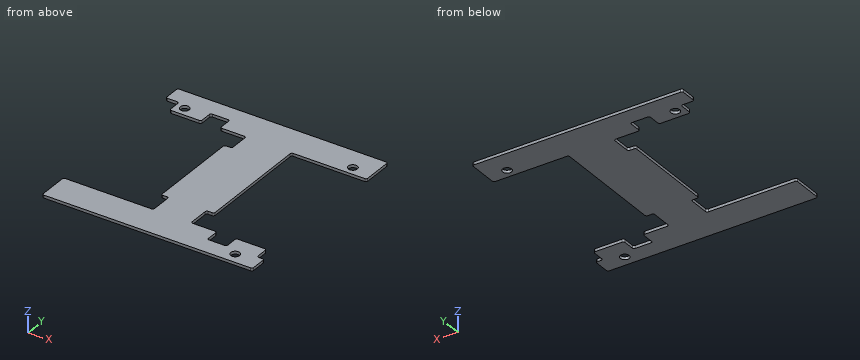
Autodesk Inventor part; units mm, degrees
ref_plane "YZ Plane" through (0, 0, 0) normal (1, 0, 0) x (0, 1, 0)
ref_plane "XZ Plane" through (0, 0, 0) normal (0, 1, 0) x (-1, 0, 0)
ref_plane "XY Plane" through (0, 0, 0) normal (0, 0, 1) x (1, 0, 0)
sketch "Sketch1" plane through (0, 0, 0) normal (0, 0, 1) x (1, 0, 0)
  line L0 (13.7023, 4) -> (22.3525, 4)
  line L1 (22.3525, 0) -> (59.3371, 0)
  line L2 (59.3371, 0) -> (59.3371, 9.3)
  line L3 (59.3371, 9.3) -> (0, 9.3)
  line L4 (0, 4) -> (0, 9.3)
  line L5 (2.4551, 0) -> (13.7023, 0)
  line L6 (0, -38.4) -> (39.318, -38.4)
  line L7 (0, -38.4) -> (0, -47.7)
  line L8 (0, -47.7) -> (59.3371, -47.7)
  line L9 (59.3371, -42.4) -> (59.3371, -47.7)
  line L10 (59.3371, -42.4) -> (58.882, -42.4)
  line L11 (58.882, -42.4) -> (58.882, -38.4)
  line L12 (47.6348, -38.4) -> (58.882, -38.4)
  line L13 (47.6348, -42.4) -> (39.318, -42.4)
  line L14 (39.0735, -33.15) -> (39.0735, -5.25)
  line L15 (39.0735, -5.25) -> (39.9371, -5.25)
  line L16 (39.9371, -5.25) -> (39.9371, -33.15)
  line L17 (39.9371, -33.15) -> (39.0735, -33.15)
  line L18 (22.2636, -5.25) -> (22.2636, -33.15)
  line L19 (22.2636, -33.15) -> (21.4, -33.15)
  line L20 (21.4, -33.15) -> (21.4, -5.25)
  line L21 (21.4, -5.25) -> (22.2636, -5.25)
  line L22 (21.4, 0) -> (21.4, -38.4)
  line L23 (39.9371, -38.4) -> (39.9371, 0)
  line L24 (39.9371, 0) -> (62.3371, 0)
  line L25 (59.1371, 9.1) -> (59.1371, 0.2)
  line L26 (59.1371, 0.2) -> (38.0735, 0.2)
  line L27 (38.0735, 0.2) -> (38.0735, -6.25)
  line L28 (38.0735, -6.25) -> (38.0735, -6.25)
  line L29 (38.0735, -6.25) -> (38.0735, -32.15)
  line L30 (35.9371, -32.15) -> (35.9371, -38.6)
  line L31 (59.1371, -42.6) -> (59.1371, -47.5)
  line L32 (59.1371, -47.5) -> (46.1371, -47.5)
  line L33 (0.2, -47.5) -> (0.2, -38.6)
  line L34 (0.2, -38.6) -> (25.4, -38.6)
  line L35 (25.4, -38.6) -> (25.4, -32.15)
  line L36 (25.4, -32.15) -> (23.2636, -32.15)
  line L37 (23.2636, -32.15) -> (23.2636, -5.75)
  line L38 (23.2636, -5.75) -> (25.4, -5.75)
  line L39 (25.4, -5.75) -> (25.4, 0.2)
  line L40 (0.2, 4.2) -> (0.2, 8.5299)
  line L41 (38.0735, -32.15) -> (35.9371, -32.15)
  line L42 (12.7424, 4.2) -> (12.7424, 0.2)
  line L43 (12.7424, 0.2) -> (3.912, 0.2)
  line L44 (3.912, 0.2) -> (3.912, 4.2)
  line L45 (3.912, 4.2) -> (0.2, 4.2)
  line L46 (59.1371, -42.6) -> (57.125, -42.6)
  line L47 (57.125, -42.6) -> (57.125, -38.6)
  line L48 (57.125, -38.6) -> (48.5947, -38.6)
  line L49 (48.5947, -38.6) -> (48.5947, -42.6)
  line L50 (39.318, -42.4) -> (39.318, -38.4)
  line L51 (47.6348, -38.4) -> (47.6348, -42.4)
  line L52 (22.3525, 4) -> (22.3525, 0)
  spline S0 degree 2 poles (41.0471, 11.3) (40.5342, 11.2191) (40.0213, 11.3) knots 0 0 0 0.102903 0.102903 0.102903 weights 1 1.01269 1
  line L53 (0, 11.3) -> (40.0213, 11.3)
  line L54 (0, 9.3) -> (0, 11.3)
  line L55 (0, 9.3) -> (46.3371, 9.3)
  line L56 (46.3371, 9.3) -> (46.3371, 11.3)
  line L57 (41.0471, 11.3) -> (46.3371, 11.3)
  spline S1 degree 2 poles (20.1962, -49.7) (20.5821, -49.6542) (20.9681, -49.7) knots 0 0 0 0.077319 0.077319 0.077319 weights 1 1.007125 1
  line L58 (46.3371, -49.7) -> (20.9681, -49.7)
  line L59 (46.3371, -47.7) -> (46.3371, -49.7)
  line L60 (0, -47.7) -> (46.3371, -47.7)
  line L61 (0, -47.7) -> (0, -49.7)
  line L62 (20.1962, -49.7) -> (0, -49.7)
  line L63 (46.1371, -47.5) -> (0.2, -47.5)
  line L64 (46.1371, -47.5) -> (46.1371, -47.5)
  line L65 (46.1371, 9.1) -> (59.1371, 9.1)
  line L66 (46.1371, 9.1) -> (46.1371, 9.1)
  line L67 (46.1371, 9.1) -> (0.2, 9.1)
  line L68 (0.2, 9.1) -> (0.2, 8.5299)
  line L69 (3.712, 4) -> (3.712, 0)
  line L70 (12.9424, 0) -> (12.9424, 4)
  line L71 (17.9365, 4) -> (17.9365, 0)
  line L72 (12.7424, 4.2) -> (18.1365, 4.2)
  line L73 (18.1365, 4.2) -> (18.1365, 0.2)
  line L74 (18.1365, 0.2) -> (25.4, 0.2)
  line L75 (43.4006, -42.4) -> (43.4006, -38.4)
  line L76 (48.3947, -38.4) -> (48.3947, -42.4)
  line L77 (57.625, -42.4) -> (57.625, -38.4)
  line L78 (35.9371, -38.6) -> (43.2006, -38.6)
  line L79 (43.2006, -38.6) -> (43.2006, -42.6)
  line L80 (43.2006, -42.6) -> (48.5947, -42.6)
  circle A0 centre (6.462, 2.75) radius 1.0065 construction
  circle A1 centre (6.462, 2.75) radius 1.25
  circle A2 centre (53.6076, 2.75) radius 1.0065 construction
  circle A3 centre (53.6076, 2.75) radius 1.25
  circle A4 centre (52.2136, -44.4) radius 1.0065 construction
  circle A5 centre (52.2136, -44.4) radius 1.25
  point P0 (0, 0)
  point P1 (38.0735, 0)
  point P2 (35.9371, -38.4)
  point P3 (52.2136, -44.4)
  dimension "d1" = 0.2
  dimension "d3" = 0.2
  dimension "d5" = 0.2
  dimension "d7" = 0.2
  dimension "d8" = 0.2
  dimension "d10" = 0.2
  dimension "d11" = 0.2
  dimension "d16" = 1
  dimension "d17" = 1
  dimension "d18" = 4
  dimension "d19" = 0.5
  dimension "d20" = 1
  dimension "d21" = 1
  dimension "d22" = 1
  dimension "d23" = 1.8636
  dimension "d24" = 4
  dimension "d25" = 4
  dimension "d35" = 0.2
  dimension "d40" = 0.2
  dimension "d42" = 0.2
  dimension "d44" = 0.2
  dimension "d47" = 0.2
  dimension "d48" = 0.2
  dimension "d50" = 0
  dimension "d51" = 0.2
  dimension "d52" = 0.2
  dimension "d53" = 0.2
  dimension "d54" = 0.2
  dimension "d55" = 0.2
  dimension "d56" = 0.2
  dimension "d57" = 0.2
  dimension "d59" = 0.2
  dimension "d60" = 0.2
  dimension "d61" = 0.2
  dimension "d62" = 0.5
  dimension "d63" = 0.2
  dimension "d64" = 0.2
  dimension "d65" = 2.5
  dimension "d66" = 2.5
  dimension "d67" = 2.5
extrude "Extrusion1" add sketch "Sketch1" along normal blind 0.8 contours L73 L72 L42 L43 L44 L45 L40 L68 L67 L65 L25 L26 L27 L1 L39 L74 L52 L0 | L0 L52 L74 L73 | L1 L27 L29 L41 L30 L6 L35 L36 L37 L38 L39 | L30 L78 L50 L13 L79 L80 L49 L48 L47 L46 L31 L32 L63 L33 L34 L35 L6 | L78 L79 L13 L50
fillet "Fillet1" radius 0.5 30 edges at (59.1371, -47.5, 0.4) (59.1371, -42.6, 0.4) (0.2, -38.6, 0.4) (25.4, -38.6, 0.4) (25.4, -32.15, 0.4) (23.2636, -32.15, 0.4) (23.2636, -5.75, 0.4) (25.4, -5.75, 0.4) (25.4, 0.2, 0.4) (0.2, 4.2, 0.4) (59.1371, 9.1, 0.4) (59.1371, 0.2, 0.4) (38.0735, 0.2, 0.4) (38.0735, -32.15, 0.4) (35.9371, -32.15, 0.4) (35.9371, -38.6, 0.4) (3.912, 4.2, 0.4) (3.912, 0.2, 0.4) (12.7424, 4.2, 0.4) (12.7424, 0.2, 0.4) (48.5947, -42.6, 0.4) (48.5947, -38.6, 0.4) (57.125, -38.6, 0.4) (57.125, -42.6, 0.4) (0.2, -47.5, 0.4) (0.2, 9.1, 0.4) (43.2006, -38.6, 0.4) (18.1365, 4.2, 0.4) (18.1365, 0.2, 0.4) (43.2006, -42.6, 0.4)
equation "\"d5\" = d1"
equation "\"d7\" = d1"
equation "\"d8\" = d1"
equation "\"d10\" = d1"
equation "\"d40\" = d1"
properties part number "PCB_InterfaceBoard"
Can you work these out from the model? Positions are in its coordinate system, mm. Give positions to 0.01 mm unless a question says otherwise; leave off trailing zeros. Write each loop counter-clockwise with the first axis right and the second up, starting at its lowest first coordinate (ties: lowest second). Pieces come first, ordered by that corner, then holes. Notation, with made-up numbers: M -26.5,29.5 L -10.5,29.5 A16 cw -10.5,57.5 Z; hole C 42,5.5 d11. An arc over 180 degrees is marked long. Answer in a Markdown table with one row per item. Add a question column.
Item 1: Imagine slicing it at C-C, the plane y = -44.4. Write out the boundary of the cut face in (x, z).
Item 2: Imagine slicing it at D-D, the plane z = 0.35. State how many separate pieces and enclosed holes the cut face has, plus the area to 3 significant figures.
Item 3: Please list where these lines run through material, in increasing order: L1, parallel to Y at x = 6.5, z = 0.6; L2, parallel to Y at x = 11.5, z = 0.1; L3, parallel to Y at x = 48, z = 0.1.
Item 4: Imagine slicing it at B-B, the plane x = 44.5. Write out the boundary of the cut face in (y, z), plus the area to 3 significant figures.
Item 5: Imagine slicing it at A-A, the plane y = 2.75. Write out the boundary of the cut face in (x, z), plus the area to 3 significant figures.
Evaluation:
| question | item | result |
|---|---|---|
| 1 | outline | M 0.2,0 L 50.96,0 L 50.96,0.8 L 0.2,0.8 Z; M 53.46,0 L 59.14,0 L 59.14,0.8 L 53.46,0.8 Z |
| 2 | separate pieces | 1 |
| 2 | enclosed holes | 3 |
| 2 | area | 1,500 mm² |
| 3 | L1 | y = -47.5 to -38.6, 0.2 to 1.5, 4 to 9.1 |
| 3 | L2 | y = -47.5 to -38.6, 0.2 to 9.1 |
| 3 | L3 | y = -47.5 to -42.6, 0.2 to 9.1 |
| 4 | outline | M -47.5,0 L -42.6,0 L -42.6,0.8 L -47.5,0.8 Z; M 0.2,0 L 9.1,0 L 9.1,0.8 L 0.2,0.8 Z |
| 4 | area | 11.0 mm² |
| 5 | outline | M 3.91,0 L 5.21,0 L 5.21,0.8 L 3.91,0.8 Z; M 7.71,0 L 12.74,0 L 12.74,0.8 L 7.71,0.8 Z; M 18.14,0 L 52.36,0 L 52.36,0.8 L 18.14,0.8 Z; M 54.86,0 L 59.14,0 L 59.14,0.8 L 54.86,0.8 Z |
| 5 | area | 35.9 mm² |
